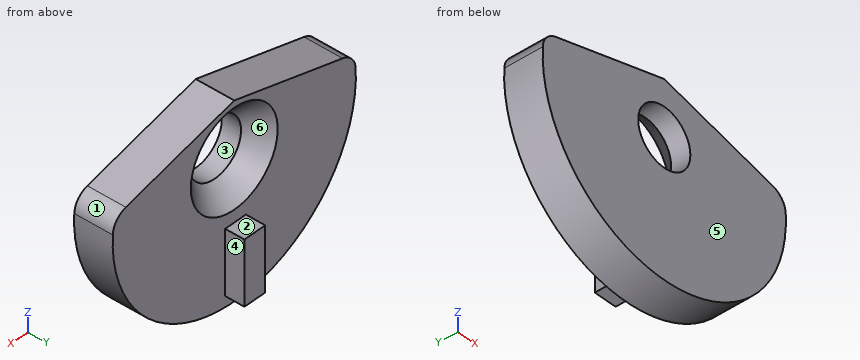
from build123d import *

# Parameters (mm, degrees)
SKETCH1_R           = 7
SKETCH1_R_2         = 1.5
BOSS_EXTRUDE1_DEPTH = 2
SKETCH2_W           = 15.705717302
SKETCH2_H           = 4.43210583
CUT_EXTRUDE1_DEPTH  = 2
CHAMFER1_SIZE       = 1
SKETCH3_W           = 1.195235373
SKETCH3_H           = 3.298389924
BOSS_EXTRUDE2_DEPTH = 1
CUT_EXTRUDE2_DEPTH  = 5
FILLET1_R           = 1


with BuildPart() as part:
    # Sketch1 → Boss-Extrude1 (new body)
    with BuildSketch(Plane(origin=(0, 0, 0), x_dir=(1, 0, 0), z_dir=(0, 1, 0))):
        with Locations((-0.805155446, -2.103263206)):
            Circle(SKETCH1_R)
        with Locations((-0.805155446, -2.103263206)):
            Circle(SKETCH1_R_2, mode=Mode.SUBTRACT)
    extrude(amount=BOSS_EXTRUDE1_DEPTH)

    # Sketch2 → Cut-Extrude1 (cut)
    with BuildSketch(Plane(origin=(0, 2, 0), x_dir=(1, 0, 0), z_dir=(0, 1, 0))):
        with Locations((-1.273649854, -7.174901084)):
            Rectangle(SKETCH2_W, SKETCH2_H)
    extrude(amount=-CUT_EXTRUDE1_DEPTH, mode=Mode.SUBTRACT)

    # Chamfer1
    chamfer1_edges = [part.edges().sort_by_distance(p)[0] for p in [
        (-2.305155446, 2, 2.103263206),
    ]]
    chamfer(chamfer1_edges, length=CHAMFER1_SIZE)

    # Sketch3 → Boss-Extrude2 (add)
    with BuildSketch(Plane(origin=(0, 2, 0), x_dir=(1, 0, 0), z_dir=(0, 1, 0))):
        with Locations((-0.879857657, 2.675462874)):
            Rectangle(SKETCH3_W, SKETCH3_H)
    extrude(amount=BOSS_EXTRUDE2_DEPTH)

    # Sketch4 → Cut-Extrude2 (cut)
    with BuildSketch(Plane(origin=(0, 2, 0), x_dir=(1, 0, 0), z_dir=(0, 1, 0))):
        Polygon((-0.805155446, -4.958848169), (-9.111708645, -2.862197678), (-9.111708645, -6.506834359), (7.404077395, -6.506834359), (7.404077395, -2.862197678), align=None)
    extrude(amount=-CUT_EXTRUDE2_DEPTH, mode=Mode.SUBTRACT)

    # Fillet1
    fillet1_edges = [part.edges().sort_by_distance(p)[0] for p in [
        (6.109528179, 1, 3.192827507),
        (-7.716407835, 1, 3.214384447),
    ]]
    fillet(fillet1_edges, radius=FILLET1_R)


solid = part.part
Source: CAD feature listing. Evaluate the final solid. Frame: model axes, mm. Face numbers are marked on the shaded views. A direction names the side the tool comes from. Round coordinates to 2 decimals unless told otherwise and drop trailing zeros. Order: outer loops, then holes, each group sorted by start corner. A loop starts at its lowest first (then second) coordinate and runs counter-clockwise, first axis right, second up. Notation, with made-up numbers: (16, -32) -> (38, -32) arc R25 ccw to (38, -6) -> close; hole circle Ø7 at (10, 85). An arc over 180 degrees is marked (long way). Answer as CSV lines item,"result".
Item 1: Section D-D, the plane x = -4.5. Return loops of the section in (y, z).
A:
outline,"(0, -3.84) -> (2, -3.84) -> (2, 4.03) -> (0, 4.03) -> close"
Item 2: Pull-direction query (X, two-part tool) for the marked faces 3, 4, 5 and 6; classes: pulls with the +X half, pulls with the -X half, needs draft (parallel to the pull), parting line crosses it, or undercut.
A:
face 3,"undercut"
face 4,"pulls with the +X half"
face 5,"needs draft"
face 6,"undercut"
Item 3: Section C-C, the plane y = 2.5. Return loops of the section in (x, z).
A:
outline,"(-1.48, -4.32) -> (-0.28, -4.32) -> (-0.28, -1.03) -> (-1.48, -1.03) -> close"
Item 4: Pin query (flat end, axial travel): pin 1 Ø2.5 at (x, z) = (-0.81, 2.1) entering from -Y; pin 2 Ø1 at (x, y) = (2, 1.5) entering from -Z; pin 3 Ø0.8 at (y, z) = (2.5, -2) entering from -X; pin 4 Ø0.8 at (y, z) = (2.5, -2.5) entering from +X. Return the tip coordinate at first contact, or that it passes through.
A:
pin 1,"through"
pin 2,"z = -4.51"
pin 3,"x = -1.48"
pin 4,"x = -0.28"
Item 5: Line query: L1, parallel to X at y = 1.55, z = 1; L2, parallel to X at y = 2.15, z = -4; L3, parallel to X at y = 1.15, z = 2.5. Output: solid intervals per line, ascending.
A:
L1,"-7.72 to -2.53, 0.92 to 6.11"
L2,"-1.48 to -0.28"
L3,"-7.79 to -2.41, 0.8 to 6.18"
Item 6: Section B-B, the plane z = -1.5. Return loops of the section in (x, y).
A:
outline,"(-6.81, 0) -> (5.2, 0) -> (5.2, 2) -> (-0.28, 2) -> (-0.28, 3) -> (-1.48, 3) -> (-1.48, 2) -> (-6.81, 2) -> close"
Item 7: Reachability of the marked faces 1 and 2 from +Z, -Z, +X, -X, +Y, -Y: full face, straight path, thin tool, end or side. Return the list, or none.
A:
face 1,"+Z, +X, +Y, -Y"
face 2,"+Z, +X, -X, +Y"
